```python
from build123d import *

# Parameters (mm, degrees)
BOSS_EXTRUDE1_DEPTH = 25
CUT_EXTRUDE7_REACH  = 80
CUT_EXTRUDE7_START  = -3
SKETCH3_R           = 3
SKETCH3_R_2         = 1.6
CUT_EXTRUDE8_REACH  = 77
SKETCH3_3_R         = 1.6
CUT_EXTRUDE9_REACH  = 80
CUT_EXTRUDE9_START  = -3
SKETCH4_R           = 3
SKETCH4_R_2         = 1.6
CUT_EXTRUDE10_REACH = 77
SKETCH4_2_R         = 1.6


with BuildPart() as part:
    # Sketch1 → Boss-Extrude1 (new body)
    with BuildSketch(Plane(origin=(0, 0, 0), x_dir=(0, 0, -1), z_dir=(1, 0, 0))):
        Polygon((0, 0), (-75, -48.70556949), (-75, -23.70556949), (0, 25), align=None)
    extrude(amount=BOSS_EXTRUDE1_DEPTH)

    # Sketch3 → Cut-Extrude7 (cut, up to next)
    with BuildSketch(Plane(origin=(0, 0, 0), x_dir=(-1, 0, 0), z_dir=(0, 0, -1)).offset(CUT_EXTRUDE7_START), mode=Mode.PRIVATE) as cut_extrude7_sk1:
        with Locations((-20, 20)):
            Circle(SKETCH3_R)
        with Locations((-20, 20)):
            Circle(SKETCH3_R_2, mode=Mode.SUBTRACT)
    cut_extrude7_tool1 = extrude(cut_extrude7_sk1.sketch, amount=-CUT_EXTRUDE7_REACH, mode=Mode.PRIVATE) & part.part
    add(cut_extrude7_tool1.solids().sort_by_distance((22.915147, 20, 3))[0], mode=Mode.SUBTRACT)
    # Sketch3 → Cut-Extrude7 (cut, up to next)
    with BuildSketch(Plane(origin=(0, 0, 0), x_dir=(-1, 0, 0), z_dir=(0, 0, -1)).offset(CUT_EXTRUDE7_START), mode=Mode.PRIVATE) as cut_extrude7_sk2:
        with Locations((-20, 5)):
            Circle(SKETCH3_R)
        with Locations((-20, 5)):
            Circle(SKETCH3_R_2, mode=Mode.SUBTRACT)
    cut_extrude7_tool2 = extrude(cut_extrude7_sk2.sketch, amount=-CUT_EXTRUDE7_REACH, mode=Mode.PRIVATE) & part.part
    add(cut_extrude7_tool2.solids().sort_by_distance((22.915147, 5, 3))[0], mode=Mode.SUBTRACT)
    # Sketch3 → Cut-Extrude7 (cut, up to next)
    with BuildSketch(Plane(origin=(0, 0, 0), x_dir=(-1, 0, 0), z_dir=(0, 0, -1)).offset(CUT_EXTRUDE7_START), mode=Mode.PRIVATE) as cut_extrude7_sk3:
        with Locations((-5, 5)):
            Circle(SKETCH3_R)
        with Locations((-5, 5)):
            Circle(SKETCH3_R_2, mode=Mode.SUBTRACT)
    cut_extrude7_tool3 = extrude(cut_extrude7_sk3.sketch, amount=-CUT_EXTRUDE7_REACH, mode=Mode.PRIVATE) & part.part
    add(cut_extrude7_tool3.solids().sort_by_distance((7.915147, 5, 3))[0], mode=Mode.SUBTRACT)
    # Sketch3 → Cut-Extrude7 (cut, up to next)
    with BuildSketch(Plane(origin=(0, 0, 0), x_dir=(-1, 0, 0), z_dir=(0, 0, -1)).offset(CUT_EXTRUDE7_START), mode=Mode.PRIVATE) as cut_extrude7_sk4:
        with Locations((-5, 20)):
            Circle(SKETCH3_R)
        with Locations((-5, 20)):
            Circle(SKETCH3_R_2, mode=Mode.SUBTRACT)
    cut_extrude7_tool4 = extrude(cut_extrude7_sk4.sketch, amount=-CUT_EXTRUDE7_REACH, mode=Mode.PRIVATE) & part.part
    add(cut_extrude7_tool4.solids().sort_by_distance((7.915147, 20, 3))[0], mode=Mode.SUBTRACT)

    # Sketch3_3 → Cut-Extrude8 (cut, up to next)
    with BuildSketch(Plane(origin=(0, 0, 0), x_dir=(-1, 0, 0), z_dir=(0, 0, -1)), mode=Mode.PRIVATE) as cut_extrude8_sk1:
        with Locations((-20, 20)):
            Circle(SKETCH3_3_R)
    cut_extrude8_tool1 = extrude(cut_extrude8_sk1.sketch, amount=-CUT_EXTRUDE8_REACH, mode=Mode.PRIVATE) & part.part
    add(cut_extrude8_tool1.solids().sort_by_distance((20, 20, 0))[0], mode=Mode.SUBTRACT)
    # Sketch3_3 → Cut-Extrude8 (cut, up to next)
    with BuildSketch(Plane(origin=(0, 0, 0), x_dir=(-1, 0, 0), z_dir=(0, 0, -1)), mode=Mode.PRIVATE) as cut_extrude8_sk2:
        with Locations((-20, 5)):
            Circle(SKETCH3_3_R)
    cut_extrude8_tool2 = extrude(cut_extrude8_sk2.sketch, amount=-CUT_EXTRUDE8_REACH, mode=Mode.PRIVATE) & part.part
    add(cut_extrude8_tool2.solids().sort_by_distance((20, 5, 0))[0], mode=Mode.SUBTRACT)
    # Sketch3_3 → Cut-Extrude8 (cut, up to next)
    with BuildSketch(Plane(origin=(0, 0, 0), x_dir=(-1, 0, 0), z_dir=(0, 0, -1)), mode=Mode.PRIVATE) as cut_extrude8_sk3:
        with Locations((-5, 5)):
            Circle(SKETCH3_3_R)
    cut_extrude8_tool3 = extrude(cut_extrude8_sk3.sketch, amount=-CUT_EXTRUDE8_REACH, mode=Mode.PRIVATE) & part.part
    add(cut_extrude8_tool3.solids().sort_by_distance((5, 5, 0))[0], mode=Mode.SUBTRACT)
    # Sketch3_3 → Cut-Extrude8 (cut, up to next)
    with BuildSketch(Plane(origin=(0, 0, 0), x_dir=(-1, 0, 0), z_dir=(0, 0, -1)), mode=Mode.PRIVATE) as cut_extrude8_sk4:
        with Locations((-5, 20)):
            Circle(SKETCH3_3_R)
    cut_extrude8_tool4 = extrude(cut_extrude8_sk4.sketch, amount=-CUT_EXTRUDE8_REACH, mode=Mode.PRIVATE) & part.part
    add(cut_extrude8_tool4.solids().sort_by_distance((5, 20, 0))[0], mode=Mode.SUBTRACT)

    # Sketch4 → Cut-Extrude9 (cut, up to next)
    with BuildSketch(Plane.XY.offset(75).offset(CUT_EXTRUDE9_START), mode=Mode.PRIVATE) as cut_extrude9_sk1:
        with Locations((5, -28.70556949)):
            Circle(SKETCH4_R)
        with Locations((5, -28.70556949)):
            Circle(SKETCH4_R_2, mode=Mode.SUBTRACT)
    cut_extrude9_tool1 = extrude(cut_extrude9_sk1.sketch, amount=-CUT_EXTRUDE9_REACH, mode=Mode.PRIVATE) & part.part
    add(cut_extrude9_tool1.solids().sort_by_distance((2.084853, -28.705569, 72))[0], mode=Mode.SUBTRACT)
    # Sketch4 → Cut-Extrude9 (cut, up to next)
    with BuildSketch(Plane.XY.offset(75).offset(CUT_EXTRUDE9_START), mode=Mode.PRIVATE) as cut_extrude9_sk2:
        with Locations((5, -43.70556949)):
            Circle(SKETCH4_R)
        with Locations((5, -43.70556949)):
            Circle(SKETCH4_R_2, mode=Mode.SUBTRACT)
    cut_extrude9_tool2 = extrude(cut_extrude9_sk2.sketch, amount=-CUT_EXTRUDE9_REACH, mode=Mode.PRIVATE) & part.part
    add(cut_extrude9_tool2.solids().sort_by_distance((2.084853, -43.705569, 72))[0], mode=Mode.SUBTRACT)
    # Sketch4 → Cut-Extrude9 (cut, up to next)
    with BuildSketch(Plane.XY.offset(75).offset(CUT_EXTRUDE9_START), mode=Mode.PRIVATE) as cut_extrude9_sk3:
        with Locations((20, -43.70556949)):
            Circle(SKETCH4_R)
        with Locations((20, -43.70556949)):
            Circle(SKETCH4_R_2, mode=Mode.SUBTRACT)
    cut_extrude9_tool3 = extrude(cut_extrude9_sk3.sketch, amount=-CUT_EXTRUDE9_REACH, mode=Mode.PRIVATE) & part.part
    add(cut_extrude9_tool3.solids().sort_by_distance((17.084853, -43.705569, 72))[0], mode=Mode.SUBTRACT)
    # Sketch4 → Cut-Extrude9 (cut, up to next)
    with BuildSketch(Plane.XY.offset(75).offset(CUT_EXTRUDE9_START), mode=Mode.PRIVATE) as cut_extrude9_sk4:
        with Locations((20, -28.70556949)):
            Circle(SKETCH4_R)
        with Locations((20, -28.70556949)):
            Circle(SKETCH4_R_2, mode=Mode.SUBTRACT)
    cut_extrude9_tool4 = extrude(cut_extrude9_sk4.sketch, amount=-CUT_EXTRUDE9_REACH, mode=Mode.PRIVATE) & part.part
    add(cut_extrude9_tool4.solids().sort_by_distance((17.084853, -28.705569, 72))[0], mode=Mode.SUBTRACT)

    # Sketch4_2 → Cut-Extrude10 (cut, up to next)
    with BuildSketch(Plane.XY.offset(75), mode=Mode.PRIVATE) as cut_extrude10_sk1:
        with Locations((5, -28.70556949)):
            Circle(SKETCH4_2_R)
    cut_extrude10_tool1 = extrude(cut_extrude10_sk1.sketch, amount=-CUT_EXTRUDE10_REACH, mode=Mode.PRIVATE) & part.part
    add(cut_extrude10_tool1.solids().sort_by_distance((5, -28.705569, 75))[0], mode=Mode.SUBTRACT)
    # Sketch4_2 → Cut-Extrude10 (cut, up to next)
    with BuildSketch(Plane.XY.offset(75), mode=Mode.PRIVATE) as cut_extrude10_sk2:
        with Locations((5, -43.70556949)):
            Circle(SKETCH4_2_R)
    cut_extrude10_tool2 = extrude(cut_extrude10_sk2.sketch, amount=-CUT_EXTRUDE10_REACH, mode=Mode.PRIVATE) & part.part
    add(cut_extrude10_tool2.solids().sort_by_distance((5, -43.705569, 75))[0], mode=Mode.SUBTRACT)
    # Sketch4_2 → Cut-Extrude10 (cut, up to next)
    with BuildSketch(Plane.XY.offset(75), mode=Mode.PRIVATE) as cut_extrude10_sk3:
        with Locations((20, -43.70556949)):
            Circle(SKETCH4_2_R)
    cut_extrude10_tool3 = extrude(cut_extrude10_sk3.sketch, amount=-CUT_EXTRUDE10_REACH, mode=Mode.PRIVATE) & part.part
    add(cut_extrude10_tool3.solids().sort_by_distance((20, -43.705569, 75))[0], mode=Mode.SUBTRACT)
    # Sketch4_2 → Cut-Extrude10 (cut, up to next)
    with BuildSketch(Plane.XY.offset(75), mode=Mode.PRIVATE) as cut_extrude10_sk4:
        with Locations((20, -28.70556949)):
            Circle(SKETCH4_2_R)
    cut_extrude10_tool4 = extrude(cut_extrude10_sk4.sketch, amount=-CUT_EXTRUDE10_REACH, mode=Mode.PRIVATE) & part.part
    add(cut_extrude10_tool4.solids().sort_by_distance((20, -28.705569, 75))[0], mode=Mode.SUBTRACT)


solid = part.part
```
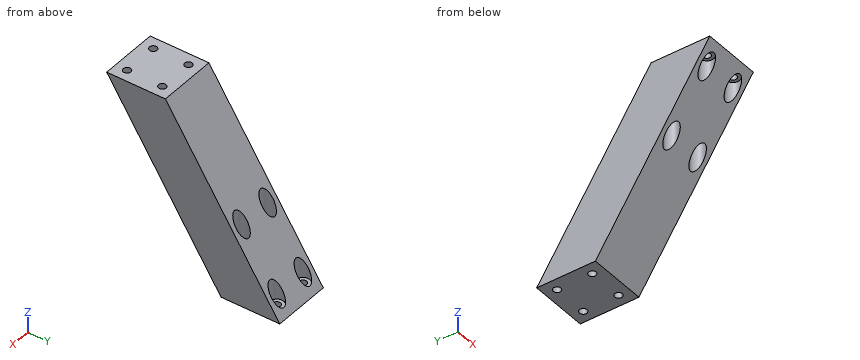
Input: part model. Units: mm. Frame: model coordinates. Round coordinates to 2 decimals unless told otherwise and drop trailing zeros. Loops run counter-clockwise (first coordinate to the right, second up) from the corner with the lowest first, then second, coordinate; pieces in that order, holes last. Notation, with made-up numbers: M -3,74 L 2,74 A5 cw 2,80 Z; hole C 66,46 d8. An arc over 180 degrees is marked long. Answer in a Markdown table with one row per item. Add a question column.
1. Contact query for flat-ended pins moving along their axis: pin 1 (8 mm diameter, centred on x = 8.5, y = 13.5, fed in from +Z); pin 2 (8 mm diameter, centred on x = 5, y = 5, fed in from +Z); pin 3 (3.5 mm diameter, centred on x = 5, y = -43.71, fed in from -Z). Output: stop coordinate, or through.
2. Section B-B (x = 9.75). Output: boundary loops of the cut face in (y, z), and give its area (4 significant figures).
3. Section A-A (y = 20). Output: boundary loops of the cut face in (x, z), and give its area (3 significant figures).
4. Ray query, probe 1 along X at (y, z) = (5, 19.5); probe 2 along Y at (x, z) = (20, 73.7); probe 3 along X at (y, z) = (-26.5, 45). Return the intervals inside material, ascending.
5. Section C-C (z = 21). Output: boundary loops of the cut face in (x, y).
6. Section D-D (y = 5). Output: boundary loops of the cut face in (x, z).
Values follow:
| question | item | result |
|---|---|---|
| 1 | pin 1 | z = 23.87 |
| 1 | pin 2 | z = 36.96 |
| 1 | pin 3 | z = 72 |
| 2 | outline | M -48.71,75 L 0,0 L 25,0 L -23.71,75 Z |
| 2 | area | 1,875 mm^2 |
| 3 | outline | M 0,0 L 3.4,0 L 3.4,3 L 2,3 L 2,7.7 L 0,7.7 Z; M 6.6,0 L 18.4,0 L 18.4,3 L 17,3 L 17,7.7 L 8,7.7 L 8,3 L 6.6,3 Z; M 21.6,0 L 25,0 L 25,7.7 L 23,7.7 L 23,3 L 21.6,3 Z |
| 3 | area | 117 mm^2 |
| 4 | probe 1 | 0 to 2, 8 to 17, 23 to 25 |
| 4 | probe 2 | -47.86 to -45.31, -42.11 to -30.31, -27.11 to -22.86 |
| 4 | probe 3 | 0 to 2.97, 7.03 to 17.97, 22.03 to 25 |
| 5 | outline | M 0,-13.64 L 25,-13.64 L 25,11.36 L 0,11.36 Z; hole C 5,5 d6; hole C 20,5 d6 |
| 6 | outline | M 0,0 L 3.4,0 L 3.4,3 L 2,3 L 2,30.8 L 0,30.8 Z; M 6.6,0 L 18.4,0 L 18.4,3 L 17,3 L 17,30.8 L 8,30.8 L 8,3 L 6.6,3 Z; M 21.6,0 L 25,0 L 25,30.8 L 23,30.8 L 23,3 L 21.6,3 Z |
